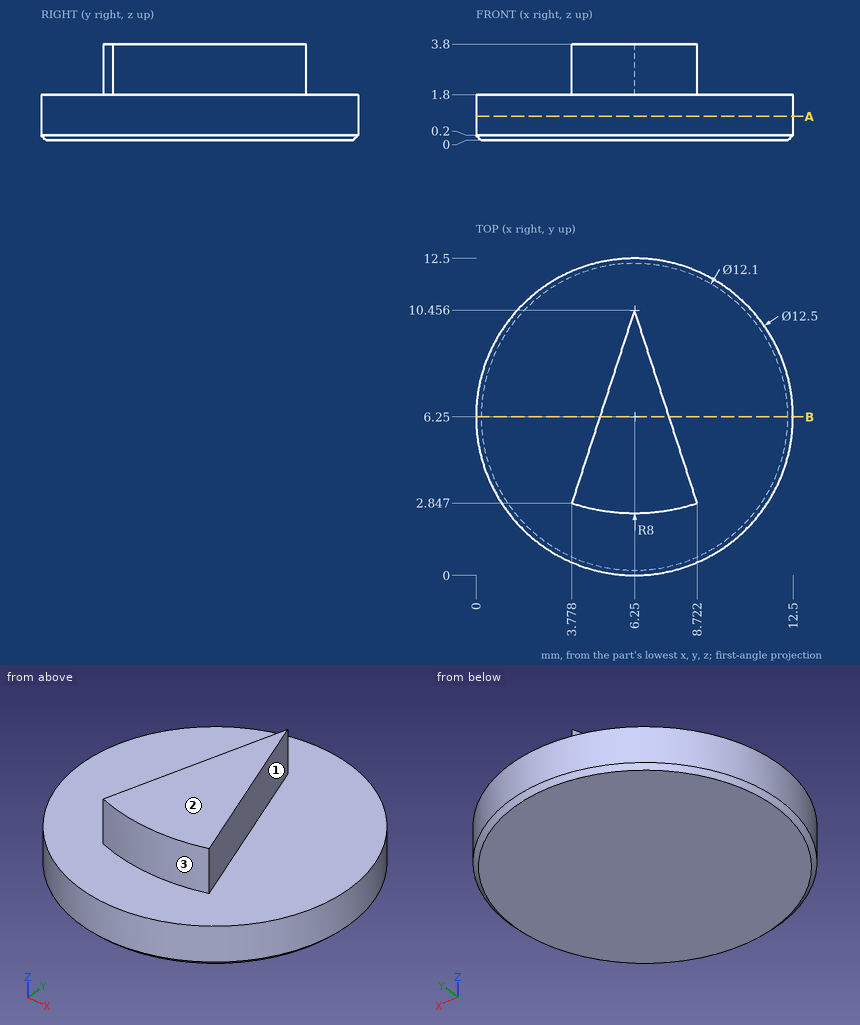
Design review of the part shown in the three views and the two pictorial views. Dimensions are in mm from the part's minimum x, y and z. A direction names the side the tool comes from. Round coordinates to 2 decimals unless told otherwise and drop trailing zeros. Loops run counter-clockwise (first coordinate to the right, second up) from the corner with the lowest first, then second, coordinate; pieces in that order, holes last. Notation, with made-up numbers: M 21.5,88 L 25.5,88 A27 cw 25.5,118 Z; hole C 23.25,11.5 d5. An arc over 180 degrees is marked long. Write item = value, one per line.
Item 1: For line 1 (Z direction, x = 1.75, y = 7); line 2 (X direction, y = 3.5, z = 2.75); line 3 (Y direction, x = 10.5, z = 1.15), list the stretches that pass through material, from the lowest coordinate up. Write a range as [from, to].
Return value:
line_1 = [0, 1.8]
line_2 = [3.99, 8.51]
line_3 = [1.67, 10.83]
Item 2: Insertion check: P1, Ø1.5, axis at y = 1.5, z = 2, coming from the -X side; P2, Ø5, axis at x = 2, y = 7, coming from the +Z side. Each pin has a flat end and moves straight along its axis. Give the tip position at first contact, or say it passes through.
Return value:
P1 = 1.47
P2 = 1.8
Item 3: Take a section at A-A on z = 0.95. Write out the cut boundary in (x, y), then the cut area to 3 significant figures.
Return value:
outline = C 6.25,6.25 d12.5
area = 123 mm2
Item 4: Machinability: for the marked faces 1, 2 and 3, which of the approach directions +Z, -Z, +X, -X, +Y, -Y give a long, thin tool a straight path to every point of the face, cutting with its end or side? Answer none if there is none.
Return value:
face_1 = +Z, +X, +Y
face_2 = +Z, +X, -X, +Y, -Y
face_3 = +Z, -Y
Item 5: Take a section at B-B on y = 6.25. Write out the cut boundary in (x, z).
Return value:
outline = M 0,0.2 L 0.2,0 L 12.3,0 L 12.5,0.2 L 12.5,1.8 L 7.62,1.8 L 7.62,3.8 L 4.88,3.8 L 4.88,1.8 L 0,1.8 Z
